Geometry check sheet. Reference: the model listing, model coordinates, mm. Face numbers are marked on the shaded views. A direction names the side the tool comes from. Coordinates: 2 decimals unless noted, no trailing zeros. Write each loop counter-clockwise with the first axis right and the second up, starting at its lowest first coordinate (ties: lowest second). Pieces come first, ordered by that corner, then holes. Notation, with made-up numbers: (40, 45.25) -> (50, 45.25) arc R12 cw to (50, 62.25) -> close; hole circle Ø3 at (23.5, 33.5). An arc over 180 degrees is marked (long way). Answer as CSV lines item,"result".
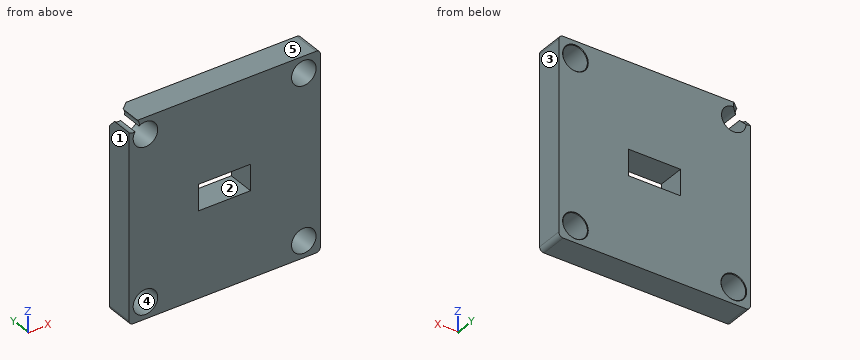
```python
from build123d import *

# Parameters (mm, degrees)
SKETCH_2_R                  = 4.5
SKETCH_2_W                  = 19
SKETCH_2_H                  = 9.5
EXTRUDE_1_DEPTH             = 10
HOLE_WIZARD_M41_D           = 4.5
HOLE_WIZARD_M41_CSINK_D     = 9.4
HOLE_WIZARD_M41_CSINK_ANGLE = 90


with BuildPart() as part:
    # Эскиз2 → Бобышка-Вытянуть1 (new body)
    with BuildSketch(Plane(origin=(0, 0, 0), x_dir=(1, 0, 0), z_dir=(0, 1, 0))):
        with BuildLine():
            Line((33.5, -36.1), (-33.5, -36.1))
            ThreePointArc((-33.5, -36.1), (-34.63137085, -35.63137085), (-35.1, -34.5))
            Line((-35.1, -34.5), (-35.1, 34.5))
            ThreePointArc((-35.1, 34.5), (-34.63137085, 35.63137085), (-33.5, 36.1))
            Line((-33.5, 36.1), (33.5, 36.1))
            ThreePointArc((33.5, 36.1), (34.63137085, 35.63137085), (35.1, 34.5))
            Line((35.1, 34.5), (35.1, -34.5))
            ThreePointArc((35.1, -34.5), (34.63137085, -35.63137085), (33.5, -36.1))
        make_face()
        with Locations(Location((-29, 30, 0), (0, 0, 270))):
            Circle(SKETCH_2_R, mode=Mode.SUBTRACT)
        with Locations(Location((29, 30, 0), (0, 0, 270))):
            Circle(SKETCH_2_R, mode=Mode.SUBTRACT)
        with Locations(Location((29, -30, 0), (0, 0, 270))):
            Circle(SKETCH_2_R, mode=Mode.SUBTRACT)
        with Locations(Location((-29, -30, 0), (0, 0, 270))):
            Circle(SKETCH_2_R, mode=Mode.SUBTRACT)
        Rectangle(SKETCH_2_W, SKETCH_2_H, mode=Mode.SUBTRACT)
    extrude(amount=EXTRUDE_1_DEPTH)

    # Зенковка для винта с полупотайной головкой M41 (through all)
    with Locations(Plane(origin=(0, 10, 0), x_dir=(1, 0, 0), z_dir=(0, 1, 0))):
        with Locations((-29, 30), (29, 30), (-33.5, -34.5), (29, -30)):
            CounterSinkHole(HOLE_WIZARD_M41_D / 2, HOLE_WIZARD_M41_CSINK_D / 2, counter_sink_angle=HOLE_WIZARD_M41_CSINK_ANGLE)


solid = part.part
```
Item 1: Cross-section at B-B, the plane z = -30. Record the cut outline in (x, y).
Responses:
outline,"(-35.1, 0) -> (-33.5, 0) -> (-33.5, 9.8) -> (-33.7, 10) -> (-35.1, 10) -> close; (-24.5, 0) -> (24.5, 0) -> (24.5, 9.8) -> (24.3, 10) -> (-24.3, 10) -> (-24.5, 9.8) -> close; (33.5, 0) -> (35.1, 0) -> (35.1, 10) -> (33.7, 10) -> (33.5, 9.8) -> close"
Item 2: Cross-section at A-A, the plane z = -0.5. Record the cut outline in (x, y), plus the area to 3 significant figures.
Responses:
outline,"(-35.1, 0) -> (-9.5, 0) -> (-9.5, 10) -> (-35.1, 10) -> close; (9.5, 0) -> (35.1, 0) -> (35.1, 10) -> (9.5, 10) -> close"
area,"512 mm2"
Item 3: Thickness scan on probe 1 along Z at (x, y) = (29, 2.5); probe 2 along X at (y, z) = (7.25, -30); probe 3 along Z at (x, y) = (-9, 7.75). Record the ranges inside material, lowest first.
Responses:
probe 1,"z = -36.1 to -34.5, -25.5 to 25.5, 34.5 to 36.1"
probe 2,"x = -35.1 to -33.5, -24.5 to 24.5, 33.5 to 35.1"
probe 3,"z = -36.1 to -4.75, 4.75 to 36.1"
Item 4: Set-up check for the marked faces 1 and 2: record each of +Z, -Z, +X, -X, +Y, -Y from which the full face is reachable in a straight line by a thin tool's end or side.
Responses:
face 1,"+Z, -Z, -X, +Y, -Y"
face 2,"+Y, -Y"
Item 5: Depth check by flat-ended pin: pin 1 Ø11.5 at (x, z) = (29, 30) entering from +Y; pin 2 Ø5.5 at (x, z) = (29, -30) entering from +Y. Enter the tip coordinate at first touch or a pass-through.
Responses:
pin 1,"stops at y = 10"
pin 2,"passes through"
Item 6: Cross-section at D-D, the plane y = 5. Record the cut outline in (x, z).
Responses:
outline,"(-35.1, -34.5) arc R1.6 ccw to (-33.5, -36.1) -> (33.5, -36.1) arc R1.6 ccw to (35.1, -34.5) -> (35.1, 34.5) arc R1.6 ccw to (33.5, 36.1) -> (-31.92, 36.1) arc R2.25 cw to (-31.35, 33.84) arc R4.5 cw (long way) to (-32.84, 32.35) arc R2.25 cw to (-35.1, 32.92) -> close; hole circle Ø9 at (-29, -30); hole (-9.5, -4.75) -> (9.5, -4.75) -> (9.5, 4.75) -> (-9.5, 4.75) -> close; hole circle Ø9 at (29, -30); hole circle Ø9 at (29, 30)"
Item 7: Release check for a two-part mould opening along X. For the marked faces 3, 4 and 5 record: +X half, -X half, draft (parallel to the pull), parting line (faces both ways), or undercut.
Responses:
face 3,"+X half"
face 4,"undercut"
face 5,"draft"
Item 8: Cross-section at C-C, the plane x = 29. Record the cut outline in (y, z), plus the area to 3 significant figures.
Responses:
outline,"(0, -36.1) -> (10, -36.1) -> (10, -34.7) -> (9.8, -34.5) -> (0, -34.5) -> close; (0, -25.5) -> (9.8, -25.5) -> (10, -25.3) -> (10, 25.3) -> (9.8, 25.5) -> (0, 25.5) -> close; (0, 34.5) -> (9.8, 34.5) -> (10, 34.7) -> (10, 36.1) -> (0, 36.1) -> close"
area,"542 mm2"
